```python
from build123d import *

# Parameters (mm, degrees)
CROQUIS1_W            = 1.5
CROQUIS1_H            = 11
CROQUIS2_R            = 3.5
CORTAR_EXTRUIR1_DEPTH = 7


with BuildPart() as part:
    # Croquis1 → Revolución1 (revolve)
    with BuildSketch(Plane.XY):
        Polygon((-13.24, -16), (-14, -16), (-14, 1.453703704), (-8.5, 4), (-4.36, 4), (-4.36, 5.5), (0, 5.5), (0, 0), (-10, 0), (-13.24, -1.5), align=None)
        with Locations((-0.75, 11)):
            Rectangle(CROQUIS1_W, CROQUIS1_H)
    revolve(axis=Axis((0, -19.446999562, 0), (0, 1, 0)))

    # Croquis2 → Cortar-Extruir1 (cut)
    with BuildSketch(Plane(origin=(0, 4, 0), x_dir=(1, 0, 0), z_dir=(0, 1, 0))):
        with Locations((0, 8.5)):
            Circle(CROQUIS2_R)
        with Locations((8.5, 0)):
            Circle(CROQUIS2_R)
        with Locations((0, -8.5)):
            Circle(CROQUIS2_R)
        with Locations((-8.5, 0)):
            Circle(CROQUIS2_R)
    extrude(amount=-CORTAR_EXTRUIR1_DEPTH, mode=Mode.SUBTRACT)


solid = part.part
```
Model file for the job. Use its own axes, mm. A direction names the side the tool comes from. Give positions to 0.01 mm unless a question says otherwise; leave off trailing zeros. Order: outer loops, then holes, each group sorted by start corner. A loop starts at its lowest first (then second) coordinate and runs counter-clockwise, first axis right, second up.
1) Mould opens along X. For faces 4 (the flat face through (0, 16.5, 0)), 5 (the conical face through (-4.045, 3.876, -7.778)), 6 (the conical face through (-9.425, -0.094, -3.908)) say: +X half, -X half, draft (parallel to the pull), parting line (faces both ways), or undercut.
2) Pin check, flat tips, straight feed: pin 1 (4 mm diameter, centred on y = -9.5, z = 6, fed in from +X); pin 2 (12 mm diameter, centred on y = 1, z = 11, fed in from -X); pin 3 (2 mm diameter, centred on x = -4, y = -2.5, fed in from -Z). Stop position of each tip, or through.
3) Saw through at B-B, the plane y = -10.5. Write the cut outline in (x, z), then the cut area to 3 significant figures.
4) Saw through at C-C, the plane y = 7. Write the cut outline in (x, z).
5) Saw through at A-A, the plane x = 0. Write the cut outline in (y, z), then the cut area to 3 significant figures.
6) Wall check: probe 1 along Z at (x, y) = (0, 0.35); probe 2 along Z at (x, y) = (0, 1.8); probe 3 along Z at (x, y) = (0, -6.5). Give the ranges that are in metal, low to high.
7) 3-axis set-ups, long thin cutter, end or side, ignore diameter. For faces 1 (the cylindrical face through (0.945, 4.76, -4.256)), 2 (the cylindrical face through (5, 2, 0)), 3 (the cylindrical face through (1.724, -8.852, 13.127)): which of +Z, -Z, +X, -X, +Y, -Y reach the whole face in a straight line?
Computed:
1. face 4: draft
1. face 5: parting line
1. face 6: undercut
2. pin 1: stops at x = 13.42
2. pin 2: stops at x = -13.08
2. pin 3: stops at z = -13.67
3. outline: circle Ø28 at (0, 0); hole circle Ø26.48 at (0, 0)
3. area: 65.0 mm2
4. outline: circle Ø3 at (0, 0)
5. outline: (-16, -14) - (1.45, -14) - (2.38, -12) - (-0.93, -12) - (-1.5, -13.24) - (-16, -13.24) - close; (-16, 13.24) - (-1.5, 13.24) - (-0.93, 12) - (2.38, 12) - (1.45, 14) - (-16, 14) - close; (0, -5) - (4, -5) - (4, -4.36) - (5.5, -4.36) - (5.5, -1.5) - (16.5, -1.5) - (16.5, 1.5) - (5.5, 1.5) - (5.5, 4.36) - (4, 4.36) - (4, 5) - (0, 5) - close
5. area: 121 mm2
6. probe 1: z = -14 to -12, -5 to 5, 12 to 14
6. probe 2: z = -13.25 to -12, -5 to 5, 12 to 13.25
6. probe 3: z = -14 to -13.24, 13.24 to 14
7. face 1: +Y
7. face 2: +Y, -Y
7. face 3: -Y
